Can you work these out from the model? Positions are in its coordinate system, mm. A direction names the side the tool comes from. Give positions to 0.01 mm unless a question says otherwise; leave off trailing zeros. Write each loop counter-clockwise with the first axis right and the second up, starting at its lowest first coordinate (ties: lowest second). Pieces come first, ordered by that corner, then holes. Notation, with made-up numbers: M 51,74.25 L 75,74.25 A18 cw 75,95.25 Z; hole C 26,30.25 d10. An arc over 180 degrees is marked long. Write each question's results on one line, items separated by ' | '.
from build123d import *

# Parameters (mm, degrees)
SKETCH1_W           = 80
SKETCH1_H           = 80
SKETCH1_R           = 4
SKETCH1_R_2         = 6
BOSS_EXTRUDE1_DEPTH = 19
SKETCH2_R           = 7
CUT_EXTRUDE1_DEPTH  = 8


with BuildPart() as part:
    # Sketch1 → Boss-Extrude1 (new body)
    with BuildSketch(Plane(origin=(0, 0, 0), x_dir=(1, 0, 0), z_dir=(0, 1, 0))):
        Rectangle(SKETCH1_W, SKETCH1_H)
        with Locations(Location((-20, 20, 0), (0, 0, 270))):
            Circle(SKETCH1_R, mode=Mode.SUBTRACT)
        with Locations(Location((20, 20, 0), (0, 0, 270))):
            Circle(SKETCH1_R, mode=Mode.SUBTRACT)
        with Locations(Location((20, -20, 0), (0, 0, 270))):
            Circle(SKETCH1_R, mode=Mode.SUBTRACT)
        with Locations(Location((-20, -20, 0), (0, 0, 270))):
            Circle(SKETCH1_R, mode=Mode.SUBTRACT)
        with Locations(Location((0, 0, 0), (0, 0, 270))):
            Circle(SKETCH1_R_2, mode=Mode.SUBTRACT)
    extrude(amount=BOSS_EXTRUDE1_DEPTH)

    # Sketch2 → Cut-Extrude1 (cut)
    with BuildSketch(Plane(origin=(0, 0, 0), x_dir=(1, 0, 0), z_dir=(0, 1, 0))):
        with Locations(Location((-20, 20, 0), (0, 0, 270))):
            Circle(SKETCH2_R)
        with Locations(Location((20, 20, 0), (0, 0, 270))):
            Circle(SKETCH2_R)
        with Locations(Location((20, -20, 0), (0, 0, 270))):
            Circle(SKETCH2_R)
        with Locations(Location((-20, -20, 0), (0, 0, 270))):
            Circle(SKETCH2_R)
    extrude(amount=CUT_EXTRUDE1_DEPTH, mode=Mode.SUBTRACT)


solid = part.part
Item 1: I'm going to push flat-ended pins straight in: pin 1 (11 mm diameter, centred on x = 0, z = 0, fed in from -Y); pin 2 (13 mm diameter, centred on x = -20, z = 20, fed in from -Y). Where does each tip first touch, or does it pass through?
Geometry says:
pin 1: passes through | pin 2: stops at y = 8
Item 2: I want a section at A-A, the plane x = 0. Please give me the cut outline in (y, z), and give its area (3 significant figures).
Geometry says:
outline: M 0,-40 L 19,-40 L 19,-6 L 0,-6 Z; M 0,6 L 19,6 L 19,40 L 0,40 Z | area: 1,290 mm2
Item 3: For faces 4 (the face through (40, 9, 1)), 5 (the face through (17, 8, -17)), which set-ups out of +Z, -Z, +X, -X, +Y, -Y let a thin tool reach every point of the face, with its end or its side?
Geometry says:
face 4: +Z, -Z, +X, +Y, -Y | face 5: -Y
Item 4: If I drill on line 1 (Z direction, x = 20, y = 14.25); line 2 (Z direction, x = -17.5, y = 1.5), over which ranges is the centre line in solid material (lowest first)? Write a range as from..to.
Geometry says:
line 1: z = -40..-24, -16..16, 24..40 | line 2: z = -40..-26.54, -13.46..13.46, 26.54..40
Item 5: I want a section at B-B, the plane z = 0. Please give me the cut outline in (x, y).
Geometry says:
outline: M -40,0 L -6,0 L -6,19 L -40,19 Z; M 6,0 L 40,0 L 40,19 L 6,19 Z
Item 6: I want a section at C-C, the plane y = 2.75. Please give me the cut outline in (x, z).
Geometry says:
outline: M -40,-40 L 40,-40 L 40,40 L -40,40 Z; hole C -20,-20 d14; hole C -20,20 d14; hole C 0,0 d12; hole C 20,-20 d14; hole C 20,20 d14
Item 7: Thinking about a two-plate mould opening in Z: for faces 1 (the face through (-1, 9, 40)), 2 (the face through (-1, 9, -40)), 3 (the face through (-16.034, 13.423, -20.521)), which applies, +Z half, -Z half, draft (parallel to the pull), parting line (faces both ways), or undercut?
Geometry says:
face 1: +Z half | face 2: -Z half | face 3: undercut
Item 8: I want a section at D-D, the plane x = 20. Please give me the cut outline in (y, z), and give its area (3 significant figures).
Geometry says:
outline: M 0,-40 L 19,-40 L 19,-24 L 8,-24 L 8,-27 L 0,-27 Z; M 0,-13 L 8,-13 L 8,-16 L 19,-16 L 19,16 L 8,16 L 8,13 L 0,13 Z; M 0,27 L 8,27 L 8,24 L 19,24 L 19,40 L 0,40 Z | area: 1,120 mm2
